from build123d import *

# Parameters (mm, degrees)
F0_R      = 20.25
F1_DEPTH  = 75
F2_SIZE2  = 49.4545935502
F2_SIZE   = 18
F3_R      = 18
F7_E11_W  = 20.25
F7_E11_H  = 50
F14_DEPTH = 1.5
F9_E17_W  = 20.25
F9_E17_H  = 50
F15_DEPTH = 1.5
F9_E13_W  = 20.25
F9_E13_H  = 50
F16_DEPTH = 1.5
F11_E21_W = 20.25
F11_E21_H = 50
F17_DEPTH = 1.5
F11_E20_W = 20.25
F11_E20_H = 50
F18_DEPTH = 1.5
F13_E23_W = 20.25
F13_E23_H = 50
F19_DEPTH = 1.5
F5_E6_W   = 20.25
F5_E6_H   = 50
F20_DEPTH = 1.5
F13_E24_W = 20.25
F13_E24_H = 50
F21_DEPTH = 1.5
F22_R     = 3.175
F22_R_2   = 2.25
F23_DEPTH = 25


with BuildPart() as f1:
    # F0 (on Top) → F1 (new body)
    with BuildSketch(Plane.XY):
        Circle(F0_R)
    extrude(amount=F1_DEPTH)

    # F2
    f2_edges = [f1.edges().sort_by_distance(p)[0] for p in [
        (-20.25, 0, 0),
    ]]
    f2_side = f1.faces().sort_by_distance((0, 0, 0))[0]
    chamfer(f2_edges, length=F2_SIZE, length2=F2_SIZE2, reference=f2_side)

    # F3
    f3_edges = [f1.edges().sort_by_distance(p)[0] for p in [
        (-20.25, 0, 75),
    ]]
    fillet(f3_edges, radius=F3_R)

    # F7_E11 (on explicit) → F14 (join, symmetric)
    with BuildSketch(Plane.YZ):
        with Locations((10.125, 25)):
            Rectangle(F7_E11_W, F7_E11_H)
    extrude(amount=F14_DEPTH, both=True)

    # F9_E17 (on explicit) → F15 (join, symmetric)
    with BuildSketch(Plane(origin=(0, 0, 0), x_dir=(-0.7071067812, 0.7071067812, 0), z_dir=(0.7071067812, 0.7071067812, 0))):
        with Locations((10.125, 25)):
            Rectangle(F9_E17_W, F9_E17_H)
    extrude(amount=F15_DEPTH, both=True)

    # F9_E13 (on explicit) → F16 (join, symmetric)
    with BuildSketch(Plane(origin=(0, 0, 0), x_dir=(-1, 0, 0), z_dir=(0, 1, 0))):
        with Locations((10.125, 25)):
            Rectangle(F9_E13_W, F9_E13_H)
    extrude(amount=F16_DEPTH, both=True)

    # F11_E21 (on explicit) → F17 (join, symmetric)
    with BuildSketch(Plane(origin=(0, 0, 0), x_dir=(-0.7071067812, -0.7071067812, 0), z_dir=(-0.7071067812, 0.7071067812, 0))):
        with Locations((10.125, 25)):
            Rectangle(F11_E21_W, F11_E21_H)
    extrude(amount=F17_DEPTH, both=True)

    # F11_E20 (on explicit) → F18 (join, symmetric)
    with BuildSketch(Plane(origin=(0, 0, 0), x_dir=(0, -1, 0), z_dir=(-1, 0, 0))):
        with Locations((10.125, 25)):
            Rectangle(F11_E20_W, F11_E20_H)
    extrude(amount=F18_DEPTH, both=True)

    # F13_E23 (on explicit) → F19 (join, symmetric)
    with BuildSketch(Plane.XZ):
        with Locations((10.125, 25)):
            Rectangle(F13_E23_W, F13_E23_H)
    extrude(amount=F19_DEPTH, both=True)

    # F5_E6 (on explicit) → F20 (join, symmetric)
    with BuildSketch(Plane(origin=(0, 0, 0), x_dir=(0.7071067812, -0.7071067812, 0), z_dir=(-0.7071067812, -0.7071067812, 0))):
        with Locations((10.125, 25)):
            Rectangle(F5_E6_W, F5_E6_H)
    extrude(amount=F20_DEPTH, both=True)

    # F13_E24 (on explicit) → F21 (join, symmetric)
    with BuildSketch(Plane(origin=(0, 0, 0), x_dir=(0.7071067812, 0.7071067812, 0), z_dir=(0.7071067812, -0.7071067812, 0))):
        with Locations((10.125, 25)):
            Rectangle(F13_E24_W, F13_E24_H)
    extrude(amount=F21_DEPTH, both=True)

    # F22 (on face) → F23 (cut)
    with BuildSketch(Plane.XY.offset(75)):
        Circle(F22_R)
        Circle(F22_R_2, mode=Mode.SUBTRACT)
        Circle(F22_R_2)
    extrude(amount=-F23_DEPTH, mode=Mode.SUBTRACT)


solid = f1.part
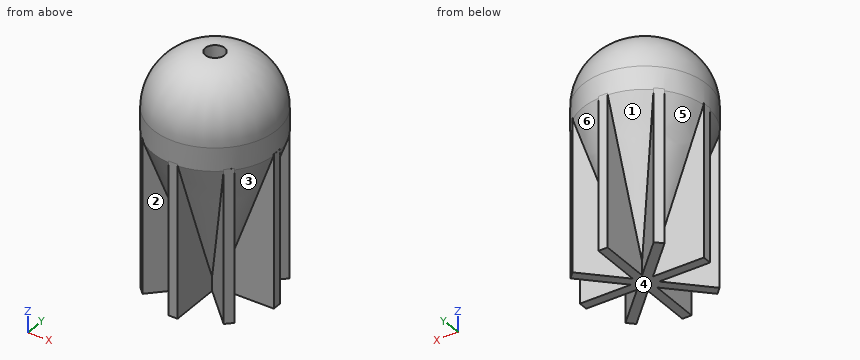
Can you work these out from the model? Positions are in its coordinate system, mm. Face numbers are marked on the shaded views. A direction names the side the tool comes from. Coordinates: 2 decimals unless noted, no trailing zeros. Answer as a JSON object with one key per item and string values. Group by question number.
Q1. Will these pins go through, and if not, where does the flat tip stop? P1, Ø4, axis at x = -6, z = 53, coming from the +Y side; P2, Ø10, axis at y = 2, z = 39, coming from the -X side; P3, Ø2, axis at x = -7, z = 26.5, coming from the +Y side; P4, Ø5, axis at y = 12, z = 14, coming from the +X side.
Q2. On a 3-axis mill with a long thin cutter (end or side, diameter ignored), from which of +Z, -Z, +X, -X, +Y, -Y can I reach the whole of each face in a straight line? I mean the marked faces 1 and 2. Say none if no direction works.
Q3. I need wall thicknesses on line 1 (Y direction, x = 0, z = 57.5) (3 decimals); line 2 (Y direction, x = -14.5, z = 8.5); line 3 (Y direction, x = 0, z = 62) (3 decimals). Which ranges of each line are inside material? Lowest first, please. Write a range as from..to.
Q4. We'd pull the mould along X, two halves only. Please class the marked faces 3, 4, 5 and 6: +X half, -X half, draft (parallel to the pull), parting line (faces both ways), or undercut.
Determined:
{
 "1": {"P1": "stops at y = 19.85", "P2": "stops at x = -20.25", "P3": "stops at y = 10.41", "P4": "stops at x = 15.38"},
 "2": {"face 1": "-Z, +Y", "face 2": "-Z, -Y"},
 "3": {"line 1": "y = -20.243..-3.175, 3.175..20.243", "line 2": "y = -14.14..-12.38, -1.5..1.5, 12.38..14.14", "line 3": "y = -19.542..-3.175, 3.175..19.542"},
 "4": {"face 3": "+X half", "face 4": "draft", "face 5": "-X half", "face 6": "undercut"}
}
